Source: CAD feature listing. Evaluate the final solid. Frame: model axes, mm. A direction names the side the tool comes from. Round coordinates to 2 decimals unless told otherwise and drop trailing zeros. Loops run counter-clockwise (first coordinate to the right, second up) from the corner with the lowest first, then second, coordinate; pieces in that order, holes last. Notation, with made-up numbers: (6.25, 1) -> (41.25, 1) arc R18 ccw to (41.25, 28) -> close; hole circle Ø11 at (-38.75, -14.5). An arc over 180 degrees is marked (long way). Write item = value, one per line.
from build123d import *

# Parameters (mm, degrees)
SKETCH1_W                = 82
SKETCH1_H                = 150
BOSS_EXTRUDE1_DEPTH      = 10
SKETCH2_W                = 10
SKETCH2_H                = 45
BOSS_EXTRUDE2_DEPTH      = 82
BOSS_EXTRUDE3_DEPTH      = 42
BOSS_EXTRUDE3_DEPTH_BACK = 10
FILLET3_RADIUS           = 26
FILLET3_LENGTH           = 10
FILLET4_RADIUS           = 26
FILLET4_LENGTH           = 10
BOSS_EXTRUDE4_DEPTH      = 10
BOSS_EXTRUDE5_DEPTH      = 10
FILLET5_R                = 15
FILLET6_R                = 15
SKETCH6_R                = 8
SKETCH6_R_2              = 5.5
CUT_EXTRUDE1_DEPTH       = 131.057679512
FILLET7_R                = 3
FILLET8_R                = 3
FILLET9_R                = 3
FILLET10_R               = 3
FILLET11_R               = 2
SKETCH7_R                = 5.5
CUT_EXTRUDE2_DEPTH       = 116.043470045
SKETCH8_W                = 182.93165677
SKETCH8_H                = 103.574339271
CUT_EXTRUDE3_DEPTH       = 131.057679512
SKETCH9_W                = 12.711196948
SKETCH9_H                = 88.540061501
BOSS_EXTRUDE6_DEPTH      = 10


with BuildPart() as part:
    # Sketch1 → Boss-Extrude1 (new body)
    with BuildSketch(Plane(origin=(0, 0, 0), x_dir=(1, 0, 0), z_dir=(0, 1, 0))):
        Rectangle(SKETCH1_W, SKETCH1_H)
    extrude(amount=BOSS_EXTRUDE1_DEPTH)

    # Sketch2 → Boss-Extrude2 (add, through all)
    with BuildSketch(Plane(origin=(41, 0, 0), x_dir=(0, 0, -1), z_dir=(1, 0, 0))):
        with Locations((70, 22.5)):
            Rectangle(SKETCH2_W, SKETCH2_H)
    extrude(amount=-BOSS_EXTRUDE2_DEPTH)

    # Sketch3 → Boss-Extrude3 (add, two sides: drawn at the far end of the back side and taken through both)
    with BuildSketch(Plane.XY.offset(-65).offset(-BOSS_EXTRUDE3_DEPTH_BACK)):
        Polygon((10, 45), (10, 10), (20, 10), (20, 45), (20, 87), (10, 87), align=None)
        Polygon((-10, 45), (-10, 87), (-20, 87), (-20, 45), (-20, 10), (-10, 10), align=None)
    extrude(amount=BOSS_EXTRUDE3_DEPTH + BOSS_EXTRUDE3_DEPTH_BACK)

    # Fillet3: full round fillet: the end face becomes a half cylinder, R = half its width
    fillet3_face = Plane((15, 87, -49), x_dir=(-1, 0, 0), z_dir=(0, 1, 0))  # on the end face: x along it, z out of the body
    fillet3_slab = fillet3_face.offset(-FILLET3_RADIUS / 2) * Box(FILLET3_LENGTH, 2 * FILLET3_RADIUS, FILLET3_RADIUS, mode=Mode.PRIVATE)  # the body's end, R deep
    fillet3_round = Plane((15, 61, -49), x_dir=(0, 1, 0), z_dir=(-1, 0, 0)) * Cylinder(FILLET3_RADIUS, FILLET3_LENGTH, mode=Mode.PRIVATE)  # its axis R under the face
    add(fillet3_slab - fillet3_round, mode=Mode.SUBTRACT)

    # Fillet4: full round fillet: the end face becomes a half cylinder, R = half its width
    fillet4_face = Plane((-15, 87, -49), x_dir=(-1, 0, 0), z_dir=(0, 1, 0))  # on the end face: x along it, z out of the body
    fillet4_slab = fillet4_face.offset(-FILLET4_RADIUS / 2) * Box(FILLET4_LENGTH, 2 * FILLET4_RADIUS, FILLET4_RADIUS, mode=Mode.PRIVATE)  # the body's end, R deep
    fillet4_round = Plane((-15, 61, -49), x_dir=(0, 1, 0), z_dir=(-1, 0, 0)) * Cylinder(FILLET4_RADIUS, FILLET4_LENGTH, mode=Mode.PRIVATE)  # its axis R under the face
    add(fillet4_slab - fillet4_round, mode=Mode.SUBTRACT)

    # Sketch4 → Boss-Extrude4 (add)
    with BuildSketch(Plane(origin=(20, 0, 0), x_dir=(0, 0, -1), z_dir=(1, 0, 0))):
        Polygon((23, 10), (23, 50), (-75, 25), (-75, 10), align=None)
    extrude(amount=-BOSS_EXTRUDE4_DEPTH)

    # Sketch5 → Boss-Extrude5 (add)
    with BuildSketch(Plane.ZY.offset(20)):
        Polygon((-23, 50), (75, 25), (75, 10), (-23, 10), align=None)
    extrude(amount=-BOSS_EXTRUDE5_DEPTH)

    # Fillet5
    fillet5_edges = [part.edges().sort_by_distance(p)[0] for p in [
        (15, 25, 75),
    ]]
    fillet(fillet5_edges, radius=FILLET5_R)

    # Fillet6
    fillet6_edges = [part.edges().sort_by_distance(p)[0] for p in [
        (-15, 25, 75),
    ]]
    fillet(fillet6_edges, radius=FILLET6_R)

    # Sketch6 → Cut-Extrude1 (cut, through all)
    with BuildSketch(Plane(origin=(20, 0, 0), x_dir=(0, 0, -1), z_dir=(1, 0, 0))):
        with Locations((49, 61)):
            Circle(SKETCH6_R)
        with Locations((-60, 17.5)):
            Circle(SKETCH6_R_2)
    extrude(amount=-CUT_EXTRUDE1_DEPTH, mode=Mode.SUBTRACT)

    # Fillet7
    fillet7_edges = [part.edges().sort_by_distance(p)[0] for p in [
        (30.5, 45, -65),
    ]]
    fillet(fillet7_edges, radius=FILLET7_R)

    # Fillet8
    fillet8_edges = [part.edges().sort_by_distance(p)[0] for p in [
        (0, 45, -65),
    ]]
    fillet(fillet8_edges, radius=FILLET8_R)

    # Fillet9
    fillet9_edges = [part.edges().sort_by_distance(p)[0] for p in [
        (-30.5, 45, -65),
    ]]
    fillet(fillet9_edges, radius=FILLET9_R)

    # Fillet10
    fillet10_edges = [part.edges().sort_by_distance(p)[0] for p in [
        (30.5, 10, -65),
        (0, 10, -65),
        (-30.5, 10, -65),
    ]]
    fillet(fillet10_edges, radius=FILLET10_R)

    # Fillet11
    fillet11_edges = [part.edges().sort_by_distance(p)[0] for p in [
        (15, 50, -23),
        (-15, 50, -23),
    ]]
    fillet(fillet11_edges, radius=FILLET11_R)

    # Sketch7 → Cut-Extrude2 (cut, through all)
    with BuildSketch(Plane(origin=(0, 10, 0), x_dir=(1, 0, 0), z_dir=(0, 1, 0))):
        with Locations(Location((31.5, 45, 0), (0, 0, 270))):
            Circle(SKETCH7_R)
        with Locations(Location((31.5, -15, 0), (0, 0, 270))):
            Circle(SKETCH7_R)
        with Locations(Location((-31.5, -15, 0), (0, 0, 90))):
            Circle(SKETCH7_R)
        with Locations(Location((-31.5, 45, 0), (0, 0, 90))):
            Circle(SKETCH7_R)
    extrude(amount=-CUT_EXTRUDE2_DEPTH, mode=Mode.SUBTRACT)

    # Sketch8 → Cut-Extrude3 (cut, through all)
    with BuildSketch(Plane.ZY.offset(20)):
        with Locations((0.186284783, 47.287847829)):
            Rectangle(SKETCH8_W, SKETCH8_H)
    extrude(amount=-CUT_EXTRUDE3_DEPTH, mode=Mode.SUBTRACT)

    # Sketch9 → Boss-Extrude6 (add, through all)
    with BuildSketch(Plane(origin=(0, 10, 0), x_dir=(1, 0, 0), z_dir=(0, 1, 0))):
        with Locations((-31.157475704, 8.108867018)):
            Rectangle(SKETCH9_W, SKETCH9_H)
    extrude(amount=-BOSS_EXTRUDE6_DEPTH)


solid = part.part
1. Section query B-B (y = 27). Return the cut outline in (x, z).
Evaluation:
outline = (-41, -75) -> (-20, -75) -> (-20, -65) -> (-41, -65) -> close
2. Section query C-C (z = -18). Return the cut outline in (x, y), then the cut area to 3 significant figures.
Evaluation:
outline = (-41, 0) -> (-20, 0) -> (-20, 10) -> (-41, 10) -> close
area = 210 mm²
3. Line query: probe 1 along Z at (x, y) = (-29.5, 38); probe 2 along Y at (x, z) = (-22.75, -57); probe 3 along Z at (x, y) = (-27, 11.5). Output: solid intervals per line, ascending. Write a range as from..to.
Evaluation:
probe_1 = -75..-65
probe_2 = 0..10
probe_3 = -75..-64.6
4. Contact query for flat-ended pins moving along their axis: pin 1 Ø6.5 at (x, z) = (-31.5, 1.5) entering from +Y; pin 2 Ø10.5 at (x, y) = (-26.5, 20.5) entering from +Z. Output: stop coordinate, or through.
Evaluation:
pin_1 = 10
pin_2 = -65
5. Set-up query: faces 1 (the face through (-31, 5, 75)), 2 (the face through (-30, 27, -65)). Return all of +Z, -Z, +X, -X, +Y, -Y with unobstructed straight access to the full face (end or side cutting, diameter ignored); none if empty.
Evaluation:
face_1 = +Z, +X, -X, +Y, -Y
face_2 = +Z, +X, -X, +Y
6. Section query A-A (x = -26). Return the cut outline in (y, z).
Evaluation:
outline = (0, -75) -> (45, -75) -> (45, -68) arc R3 ccw to (42, -65) -> (13, -65) arc R3 cw to (10, -62) -> (10, 75) -> (0, 75) -> close
